For this review, take the finished solid that the model builds, in its own axes (mm). A direction names the side the tool comes from. Round coordinates to 2 decimals unless told otherwise and drop trailing zeros. Order: outer loops, then holes, each group sorted by start corner. A loop starts at its lowest first (then second) coordinate and runs counter-clockwise, first axis right, second up. Notation, with made-up numbers: M 34,31 L 41,31 A24 cw 41,55 Z; hole C 88,39.5 d10. An arc over 180 degrees is marked long. Answer as a JSON object with one key per item and string values.
from build123d import *

# Parameters (mm, degrees)
SKETCH1_R           = 10
EXTRUDE1_DEPTH      = 45
FILLET1_R           = 4
SKETCH2_W           = 7.044053374
SKETCH2_H           = 25.342236328
SKETCH2_W_2         = 7
SKETCH2_H_2         = 23.94716261
EXTRUDE2_DEPTH      = 20
SKETCH5_W           = 5.258419436
SKETCH5_H           = 20.959398048
EXTRUDE4_DEPTH      = 48.169905777
SKETCH11_W          = 21.968744981
SKETCH11_H          = 5.630856805
EXTRUDE10_DEPTH     = 47.786750374
SKETCH12_R          = 1.5
EXTRUDE11_DEPTH     = 49.183163121
SKETCH13_R          = 1.5
EXTRUDE12_DEPTH     = 49.183163121
CHAMFER_1_SIZE      = 3
CHAMFER_1_SIZE2     = 5.196152423
SKETCH_1_R          = 1
CUT_EXTRUDE_1_DEPTH = 34.908314691


with BuildPart() as part:
    # Sketch1 → Extrude1 (new body)
    with BuildSketch(Plane(origin=(0, 0, 0), x_dir=(1, 0, 0), z_dir=(0, 1, 0))):
        with Locations(Location((0, 0, 0), (0, 0, 90))):
            Circle(SKETCH1_R)
    extrude(amount=EXTRUDE1_DEPTH)

    # Fillet1
    fillet1_edges = [part.edges().sort_by_distance(p)[0] for p in [
        (0, 0, 10),
        (0, 45, 10),
    ]]
    fillet(fillet1_edges, radius=FILLET1_R)

    # Sketch2 → Extrude2 (cut, symmetric)
    with BuildSketch(Plane.XY):
        Rectangle(SKETCH2_W, SKETCH2_H)
        with Locations((0, 42.838233159)):
            Rectangle(SKETCH2_W_2, SKETCH2_H_2)
    extrude(amount=EXTRUDE2_DEPTH, both=True, mode=Mode.SUBTRACT)

    # Sketch5 → Extrude4 (cut, through all)
    with BuildSketch(Plane(origin=(0, 0, 0), x_dir=(1, 0, 0), z_dir=(0, 1, 0))):
        with Locations((10.629209718, 0.450601309)):
            Rectangle(SKETCH5_W, SKETCH5_H)
        with Locations((-10.629209718, 0.450601309)):
            Rectangle(SKETCH5_W, SKETCH5_H)
    extrude(amount=EXTRUDE4_DEPTH, mode=Mode.SUBTRACT)

    # Sketch11 → Extrude10 (cut, through all)
    with BuildSketch(Plane(origin=(0, 45, 0), x_dir=(1, 0, 0), z_dir=(0, 1, 0))):
        with Locations((-0.154491877, -9.18859048)):
            Rectangle(SKETCH11_W, SKETCH11_H)
        with Locations((-0.154491877, 9.18859048)):
            Rectangle(SKETCH11_W, SKETCH11_H)
    extrude(amount=-EXTRUDE10_DEPTH, mode=Mode.SUBTRACT)

    # Sketch12 → Extrude11 (cut, through all)
    with BuildSketch(Plane.ZY.offset(8)):
        with Locations(Location((0, 39.462335046, 0), (0, 0, 180))):
            Circle(SKETCH12_R)
    extrude(amount=-EXTRUDE11_DEPTH, mode=Mode.SUBTRACT)

    # Sketch13 → Extrude12 (cut, through all)
    with BuildSketch(Plane.ZY.offset(8)):
        with Locations(Location((-3.026564036, 4.561005479, 0), (0, 0, 180))):
            Circle(SKETCH13_R)
        Polygon((6.818378582, 17.003077145), (-1.791354285, 0), (6.818378582, 0), align=None)
    extrude(amount=-EXTRUDE12_DEPTH, mode=Mode.SUBTRACT)

    # Фаска1
    chamfer_1_edges = [part.edges().sort_by_distance(p)[0] for p in [
        (0, 30.864651854, 6.373162077),
    ]]
    chamfer_1_side = [part.faces().sort_by_distance(p)[0] for p in [
        (0, 28.01207475, 6.373162077),
    ]]
    chamfer(chamfer_1_edges, length=CHAMFER_1_SIZE, length2=CHAMFER_1_SIZE2, reference=chamfer_1_side[0])

    # Эскиз1 → Вырез-Вытянуть1 (cut, through all)
    with BuildSketch(Plane.XZ.offset(-12.671118164)):
        with Locations(Location((-0.022026687, 3.547657951, 0), (0, 0, 270))):
            Circle(SKETCH_1_R)
    extrude(amount=-CUT_EXTRUDE_1_DEPTH, mode=Mode.SUBTRACT)


solid = part.part
1) Machinability: for faces 4 (the flat face through (3.522, 8, -2)), 5 (the cylindrical face through (5.719, 40.927, 0.325)), 6 (the flat face through (0.05, 28.72, 4.89)), which of the approach directions +Z, -Z, +X, -X, +Y, -Y give a long, thin tool a straight path to every point of the face, cutting with its end or side? Answer none if there is none.
Geometry check:
{"face 4": "+Z, -Z, -Y", "face 5": "+X, -X", "face 6": "+Z, +Y"}
2) Mouldability with a two-part tool opening along X and no side actions: class faces 1 (the flat face through (-8, 22, 0)), 2 (the flat face through (-3.522, 8, -2)), 3 (the flat face through (8, 22, 0)) as +X half, -X half, draft (parallel to the pull), parting line (faces both ways), or undercut.
Geometry check:
{"face 1": "-X half", "face 2": "undercut", "face 3": "+X half"}
3) Add section A-A on y = 37.5. State the section outline as (x, z) points.
Geometry check:
{"outline": "M -8,-6 A10 ccw -7.71,-6.37 L -3.5,-6.37 L -3.5,6.37 L -7.71,6.37 A10 ccw -8,6 Z; M 3.5,-6.37 L 7.71,-6.37 A10 ccw 8,-6 L 8,6 A10 ccw 7.71,6.37 L 3.5,6.37 Z"}
4) Add section D-D on y = 14.5. State the section outline as (x, z) points, and give its area (3 significant figures).
Geometry check:
{"outline": "M -8,-6 A10 ccw -7.71,-6.37 L 7.71,-6.37 A10 ccw 8,-6 L 8,5.55 L -8,5.55 Z; hole C -0.02,3.55 d2", "area": "188 mm²"}
5) Insertion check: P1, Ø3.5, axis at y = 39.46, z = 0, coming from the -X side. The pin has a flat end and moves straight along its axis. Give the tip position at first contact, or say it passes through.
Geometry check:
{"P1": "stops at x = -8"}
6) Add section B-B on z = 0. State the section outline as (x, y) points, and give its area (3 significant figures).
Geometry check:
{"outline": "M -8,3.54 L -3.52,3.54 L -3.52,12.67 L 3.52,12.67 L 3.52,3.54 L 8,3.54 L 8,37.96 L 3.5,37.96 L 3.5,30.86 L -3.5,30.86 L -3.5,37.96 L -8,37.96 Z; M -8,40.96 L -3.5,40.96 L -3.5,45 L -6,45 A4 ccw -8,44.46 Z; M 3.5,40.96 L 8,40.96 L 8,44.46 A4 ccw 6,45 L 3.5,45 Z", "area": "472 mm²"}
7) For L1, parallel to X at y = 43.5, z = 0; L2, parallel to Y at x = 5.5, z = 0; L3, parallel to X at y = 17, z = 3, list the stretches that pass through material, from the lowest coordinate up.
Geometry check:
{"L1": "x = -8 to -3.5, 3.5 to 8", "L2": "y = 3.54 to 37.96, 40.96 to 45", "L3": "x = -8 to -0.86, 0.81 to 8"}
8) Add section C-C on x = 0.5. State the section outline as (y, z) points.
Geometry check:
{"outline": "M 12.67,-6.37 L 30.86,-6.37 L 30.86,1.18 L 29.99,2.69 L 12.67,2.69 Z; M 12.67,4.4 L 29,4.4 L 27.86,6.37 L 16.12,6.37 L 12.67,4.62 Z"}
